```python
from build123d import *

# Parameters (mm, degrees)
BOSS_EXTRUDE1_DEPTH                 = 20
SKETCH4_R                           = 29
CUT_EXTRUDE1_DEPTH                  = 46.345892868
CHAMFER1_SIZE                       = 5
SKETCH5_W                           = 5.5
SKETCH5_H                           = 3
CUT_EXTRUDE2_DEPTH                  = 3
CUT_EXTRUDE2_DIRECTION_2_REACH      = 42.755
CUT_EXTRUDE2_DIRECTION_2_END_RADIUS = 29
SKETCH7_R                           = 1.8
CUT_EXTRUDE3_DEPTH                  = 6


with BuildPart() as part:
    # Sketch3 → Boss-Extrude1 (new, symmetric)
    with BuildSketch(Plane.XY):
        with BuildLine():
            Line((-27.5, -30), (27.5, -30))
            Line((27.5, -30), (27.5, 0))
            Line((27.5, 0), (21, 0))
            ThreePointArc((21, 0), (0, -21), (-21, 0))
            Line((-21, 0), (-27.5, 0))
            Line((-27.5, 0), (-27.5, -30))
        make_face()
    extrude(amount=BOSS_EXTRUDE1_DEPTH, both=True)

    # Sketch4 → Cut-Extrude1 (cut, through all)
    with BuildSketch(Plane(origin=(0, 0, 0), x_dir=(1, 0, 0), z_dir=(0, 1, 0))):
        with Locations((-40, 0)):
            Circle(SKETCH4_R)
        with Locations((40, 0)):
            Circle(SKETCH4_R)
    extrude(amount=-CUT_EXTRUDE1_DEPTH, mode=Mode.SUBTRACT)

    # Chamfer1
    # the kernel refuses this chamfer: 5 mm, written as the material it takes off along each edge
    with BuildSketch(Plane(origin=(0, 0, 20), x_dir=(0.9851003883005318, 0.1719803040180515, 0), z_dir=(-0.1719803040180515, 0.9851003883005318, 0))) as chamfer1_piece_1:
        Polygon((21 + CHAMFER1_SIZE, 0), (21, CHAMFER1_SIZE), (21, 0), align=None)
    revolve(axis=Axis((0, 0, 20), (0, 0, -1)), revolution_arc=199.805956235, mode=Mode.SUBTRACT)
    with BuildSketch(Plane(origin=(0, 0, -20), x_dir=(0.9851003883005321, 0.1719803040180491, 0), z_dir=(-0.1719803040180491, 0.9851003883005321, 0))) as chamfer1_piece_2:
        Polygon((21 + CHAMFER1_SIZE, 0), (21, -CHAMFER1_SIZE), (21, 0), align=None)
    revolve(axis=Axis((0, 0, -20), (0, 0, -1)), revolution_arc=199.805956235, mode=Mode.SUBTRACT)

    # Sketch5 → Cut-Extrude2 (cut)
    with BuildSketch(Plane(origin=(0, 0, 0), x_dir=(0, 0, -1), z_dir=(1, 0, 0))):
        with Locations((-12.5, -25.5)):
            Rectangle(SKETCH5_W, SKETCH5_H)
        with Locations((12.5, -25.5)):
            Rectangle(SKETCH5_W, SKETCH5_H)
    extrude(amount=-CUT_EXTRUDE2_DEPTH, mode=Mode.SUBTRACT)

    # Cut-Extrude2 direction 2: up to this cylinder (the profile starts outside it)
    cut_extrude2_direction_2_end = Plane(origin=(40, -25.5, 0), z_dir=(0, 1, 0)) * Cylinder(CUT_EXTRUDE2_DIRECTION_2_END_RADIUS, 144.51, mode=Mode.PRIVATE)
    # Sketch5 → Cut-Extrude2 direction 2 (cut, up to the surface)
    with BuildSketch(Plane(origin=(0, 0, 0), x_dir=(0, 0, -1), z_dir=(1, 0, 0)), mode=Mode.PRIVATE) as cut_extrude2_direction_2_sk1:
        with Locations((-12.5, -25.5)):
            Rectangle(SKETCH5_W, SKETCH5_H)
    cut_extrude2_direction_2_tool1 = extrude(cut_extrude2_direction_2_sk1.sketch, amount=CUT_EXTRUDE2_DIRECTION_2_REACH, mode=Mode.PRIVATE) - cut_extrude2_direction_2_end
    add(cut_extrude2_direction_2_tool1.solids().sort_by_distance((0, -25.5, 12.5))[0], mode=Mode.SUBTRACT)
    # Sketch5 → Cut-Extrude2 direction 2 (cut, up to the surface)
    with BuildSketch(Plane(origin=(0, 0, 0), x_dir=(0, 0, -1), z_dir=(1, 0, 0)), mode=Mode.PRIVATE) as cut_extrude2_direction_2_sk2:
        with Locations((12.5, -25.5)):
            Rectangle(SKETCH5_W, SKETCH5_H)
    cut_extrude2_direction_2_tool2 = extrude(cut_extrude2_direction_2_sk2.sketch, amount=CUT_EXTRUDE2_DIRECTION_2_REACH, mode=Mode.PRIVATE) - cut_extrude2_direction_2_end
    add(cut_extrude2_direction_2_tool2.solids().sort_by_distance((0, -25.5, -12.5))[0], mode=Mode.SUBTRACT)

    # Sketch7 → Cut-Extrude3 (cut)
    with BuildSketch(Plane.XZ.offset(30)):
        with Locations(Location((0, 12.5, 0), (0, 0, 270))):
            Circle(SKETCH7_R)
        with Locations(Location((0, -12.5, 0), (0, 0, 90))):
            Circle(SKETCH7_R)
    extrude(amount=-CUT_EXTRUDE3_DEPTH, mode=Mode.SUBTRACT)


solid = part.part
```
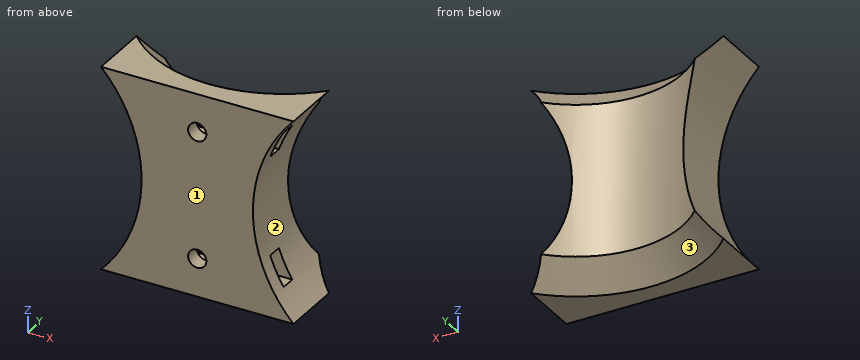
CAD build for the part. Positions are in the model's coordinates, mm. Face numbers are marked on the shaded views. Coordinates: 2 decimals unless noted, no trailing zeros. Write each loop counter-clockwise with the first axis right and the second up, starting at its lowest first coordinate (ties: lowest second). Pieces come first, ordered by that corner, then holes. Notation, with made-up numbers: (-0.75, 68.5) -> (11.25, 68.5) arc R4 ccw to (11.25, 74.5) -> close; hole circle Ø2 at (45, -30.5). An arc over 180 degrees is marked (long way). Return JSON: item names as keys, results as strings. Group by question number.
Q1. Cut at C-C, the plane x = 0. Give the cut face in (y, z), then the cut area to 3 significant figures.
Q2. Cut at B-B, the plane y = -28.5. Give the cut face in (x, z).
Q3. Cut at A-A, the plane z = 13.5. Give the cut face in (x, y).
Q4. Pull direction Z, two halves, no side cores. Call the marked faces 1, 2 and 3: released by +Z, released by -Z, zero draft, split by the parting line, or undercut.
Q5. Flat gauge pins, fed straight in: pin 1 (0.9 mm diameter, centred on y = -26, z = 12, fed in from +X); pin 2 (3.5 mm diameter, centred on x = 7, y = -25, fed in from -Z); pin 3 (1.5 mm diameter, centred on x = 3, z = 6, fed in from +Y); pin 4 (3 mm diameter, centred on x = 4, z = 12.5, fed in from +Y). Where does each tip first touch, or does it go through?
Q6. Drill centre lines: line 1 (X direction, y = -18.5, z = -14); line 2 (X direction, y = -18, z = -10); line 3 (Z direction, x = -14.5, y = -25.75). Where is each one in solid material? Low to high.
Returned:
{
 "1": {"outline": "(-30, -20) -> (-26, -20) -> (-21, -15) -> (-21, 15) -> (-26, 20) -> (-30, 20) -> (-30, 14.3) -> (-27, 14.3) -> (-27, 15.25) -> (-24, 15.25) -> (-24, 9.75) -> (-27, 9.75) -> (-27, 10.7) -> (-30, 10.7) -> (-30, -10.7) -> (-27, -10.7) -> (-27, -9.75) -> (-24, -9.75) -> (-24, -15.25) -> (-27, -15.25) -> (-27, -14.3) -> (-30, -14.3) -> close", "area": "280 mm2"},
 "2": {"outline": "(-19, -20) -> (19, -20) arc R29 cw to (19, 20) -> (-19, 20) arc R29 cw to start; hole circle Ø3.6 at (0, -12.5); hole circle Ø3.6 at (0, 12.5)"},
 "3": {"outline": "(-14.33, -30) -> (-1.5, -30) -> (-1.5, -27) -> (-3, -27) -> (-3, -24) -> (14.33, -24) -> (14.33, -15.35) arc R21 cw to (-14.33, -15.35) -> close; (1.5, -30) -> (14.33, -30) -> (14.33, -27) -> (1.5, -27) -> close"},
 "4": {"face 1": "zero draft", "face 2": "undercut", "face 3": "released by -Z"},
 "5": {"pin 1": "stops at x = -3", "pin 2": "stops at z = -20", "pin 3": "stops at y = -20.66", "pin 4": "stops at y = -20.27"},
 "6": {"line 1": "x = -14.6 to -9.94, 9.94 to 14.6", "line 2": "x = -12.78 to -10.82, 10.82 to 12.78", "line 3": "z = -20 to -13.81, 13.81 to 20"}
}
